Here's how the part is built. I have some questions about the finished solid (model axes, mm). A direction names the side the tool comes from. Coordinates: 2 decimals unless noted, no trailing zeros. Loops run counter-clockwise (first coordinate to the right, second up) from the corner with the lowest first, then second, coordinate; pieces in that order, holes last. Notation, with made-up numbers: (-7, 15) -> (9, 15) arc R15 ccw to (9, 37) -> close; hole circle Ø11 at (1.5, -40). An arc over 180 degrees is marked (long way). Answer as a JSON object with one key per item and string values. Group by question number.
1) I want a section at D-D (x = -18). Write out the boundary of the cut face in (y, z).
2) I'm going to push flat-ended pins straight in: pin 1 (8 mm diameter, centred on y = -20, z = -53, fed in from +X); pin 2 (10 mm diameter, centred on y = -14, z = -35, fed in from -X); pin 3 (12 mm diameter, centred on x = 13, z = -75.5, fed in from +Y); pin 4 (5 mm diameter, centred on x = 25.5, y = -18, fed in from -Z). Where does each tip first touch, or does it pass through?
3) Which directions (+Z, -Z, +X, -X, +Y, -Y) give clear straight access to the entire face, cutting with the end or side of a thin tool? Please do faces 1 (the flat face through (-3, -33, 0)), 2 (the flat face through (0, -35, -51)), 3 (the cylindrical face through (-18.46, -29.53, -6.34)), 4 (the flat face through (18, -33, -87.5)), 5 (the cylindrical face through (-0.681, -31.995, -50.7)).
4) If we mould it in two halves opening along X, with no side actions, what happens to faces 6 (the cylindrical face through (-0.81, -42.492, -50.7)), 7 (the flat face through (-18, -33, -87.5)), 8 (the flat face through (-3, -33, -100))? For each: +X half, -X half, draft (parallel to the pull), parting line (faces both ways), or undercut.
5) I want a section at A-A (y = -14). Write out the boundary of the cut face in (x, z), then the cut area to 3 significant figures.
6) I need wall thicknesses on probe 1 along Y at (x, z) = (-1, -76); probe 2 along X at (y, z) = (-33, -5.75); probe 3 along Y at (x, z) = (-18, -93.5). Which ranges of each line are inside material? Lowest first, please. Write a range as [from, to].
7) I want a section at C-C (z = -9). Count the separate pieces of the cut face and the enclosed holes in it, then the cut area to 3 significant figures.
8) I want a section at B-B (x = -1.5). Write out the boundary of the cut face in (y, z) (3 decimals), then the cut area to 3 significant figures.
```python
from build123d import *

# Parameters (mm, degrees)
CYLINDER017_R     = 3.5
CYLINDER017_DEPTH = 25
CYLINDER016_R     = 3.5
CYLINDER016_DEPTH = 25
CYLINDER009_R     = 3.5
CYLINDER009_DEPTH = 25
CYLINDER007_R     = 3.5
CYLINDER007_DEPTH = 25
BOX001_W          = 19
BOX001_H          = 4
BOX001_DEPTH      = 100
CYLINDER002_R     = 45
CYLINDER002_DEPTH = 100
CYLINDER003_R     = 42.5
CYLINDER003_DEPTH = 100
FILLET003_R       = 1
FILLET002_R       = 1


with BuildPart() as cylindre015:
    # Cylinder017 → Cylinder017 (new body)
    with BuildSketch(Plane(origin=(18, -33, -112.5), x_dir=(1, 0, 0), z_dir=(0, 0, 1))):
        Circle(CYLINDER017_R)
    extrude(amount=CYLINDER017_DEPTH)


with BuildPart() as cylindre014:
    # Cylinder016 → Cylinder016 (new body)
    with BuildSketch(Plane(origin=(-18, -33, -112.5), x_dir=(1, 0, 0), z_dir=(0, 0, 1))):
        Circle(CYLINDER016_R)
    extrude(amount=CYLINDER016_DEPTH)


with BuildPart() as cylindre009:
    # Cylinder009 → Cylinder009 (new body)
    with BuildSketch(Plane(origin=(18, -33, -12.5), x_dir=(1, 0, 0), z_dir=(0, 0, 1))):
        Circle(CYLINDER009_R)
    extrude(amount=CYLINDER009_DEPTH)


with BuildPart() as cylindre007:
    # Cylinder007 → Cylinder007 (new body)
    with BuildSketch(Plane(origin=(-18, -33, -12.5), x_dir=(1, 0, 0), z_dir=(0, 0, 1))):
        Circle(CYLINDER007_R)
    extrude(amount=CYLINDER007_DEPTH)


with BuildPart() as cube001:
    # Box001 → Box001 (new body)
    with BuildSketch(Plane(origin=(-9.5, -39, 0), x_dir=(1, 0, 0), z_dir=(0, 0, 1))):
        with Locations((9.5, 2)):
            Rectangle(BOX001_W, BOX001_H)
    extrude(amount=BOX001_DEPTH)


with BuildPart() as cylindre002:
    # Cylinder002 → Cylinder002 (new body)
    with BuildSketch(Plane(origin=(0, 13, 0), x_dir=(1, 0, 0), z_dir=(0, 0, 1))):
        Circle(CYLINDER002_R)
    extrude(amount=CYLINDER002_DEPTH)


with BuildPart() as cut011:
    # Cylinder003 → Cylinder003 (new body)
    with BuildSketch(Plane.XY):
        Circle(CYLINDER003_R)
    extrude(amount=CYLINDER003_DEPTH)

    # Cut003: cut Cylindre002
    add(cylindre002.part, mode=Mode.SUBTRACT)

    # Fillet003
    fillet003_edges = [cut011.edges().sort_by_distance(p)[0] for p in [
        (-42.456904, -1.913462, 50),
    ]]
    fillet(fillet003_edges, radius=FILLET003_R)

    # Fillet002
    fillet002_edges = [cut011.edges().sort_by_distance(p)[0] for p in [
        (42.456904, -1.913462, 50),
    ]]
    fillet(fillet002_edges, radius=FILLET002_R)

    # Cut002: cut Cube001
    add(cube001.part, mode=Mode.SUBTRACT)


with BuildPart() as cut011_1:
    # Cut002 placement: moved
    add(cut011.part.moved(Location((0, 0, -100))))

    # Cut007: cut Cylindre007
    add(cylindre007.part, mode=Mode.SUBTRACT)

    # Cut008: cut Cylindre009
    add(cylindre009.part, mode=Mode.SUBTRACT)

    # Cut010: cut Cylindre014
    add(cylindre014.part, mode=Mode.SUBTRACT)

    # Cut011: cut Cylindre015
    add(cylindre015.part, mode=Mode.SUBTRACT)


solid = cut011_1.part
```
Determined:
{
 "1": {"outline": "(-38.5, -100) -> (-36.5, -100) -> (-36.5, -87.5) -> (-29.5, -87.5) -> (-29.5, -100) -> (-28.24, -100) -> (-28.24, 0) -> (-29.5, 0) -> (-29.5, -12.5) -> (-36.5, -12.5) -> (-36.5, 0) -> (-38.5, 0) -> close"},
 "2": {"pin 1": "x = 39.37", "pin 2": "x = -41.54", "pin 3": "y = -27.79", "pin 4": "through"},
 "3": {"face 1": "+Z, +X, -X, +Y, -Y", "face 2": "+Z, -Z", "face 3": "+Z", "face 4": "-Z", "face 5": "+Z, -Z, +Y"},
 "4": {"face 6": "parting line", "face 7": "undercut", "face 8": "draft"},
 "5": {"outline": "(-40.13, -100) -> (-36, -100) -> (-36, 0) -> (-40.13, 0) -> close; (36, -100) -> (40.13, -100) -> (40.13, 0) -> (36, 0) -> close", "area": "826 mm^2"},
 "6": {"probe 1": "[-42.49, -39], [-35, -31.99]", "probe 2": "[-26.78, -21.5], [-14.5, 14.5], [21.5, 26.78]", "probe 3": "[-38.5, -36.5], [-29.5, -28.24]"},
 "7": {"separate pieces": "1", "enclosed holes": "3", "area": "647 mm^2"},
 "8": {"outline": "(-42.474, -100) -> (-39, -100) -> (-39, 0) -> (-42.474, 0) -> close; (-35, -100) -> (-31.975, -100) -> (-31.975, 0) -> (-35, 0) -> close", "area": "650 mm^2"}
}
